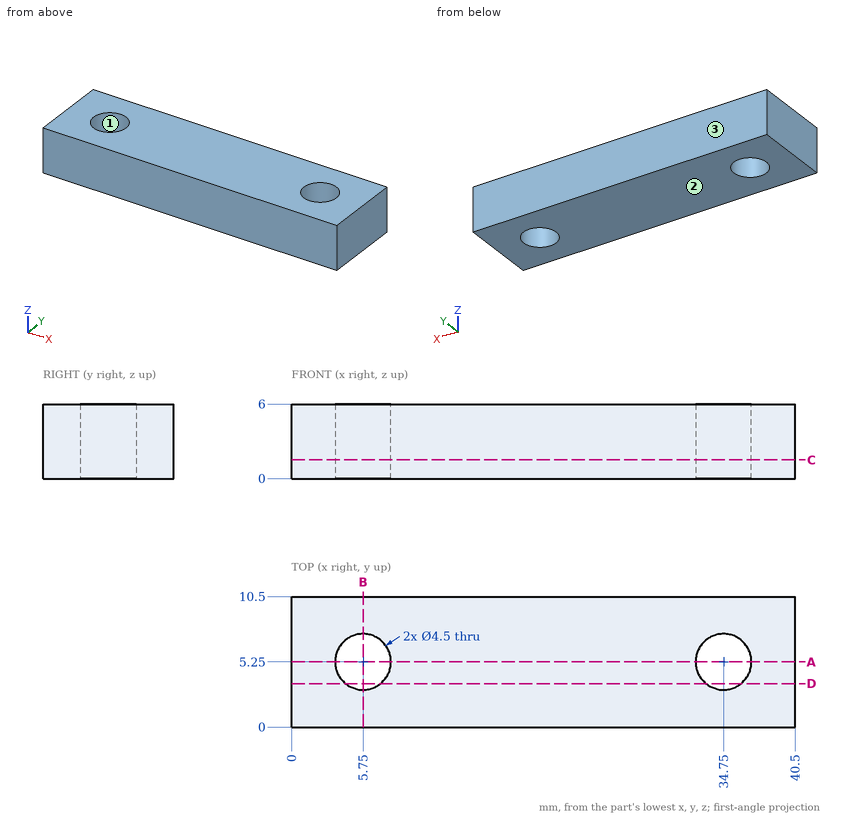
Could you check a few things on this drawing? It's one solid part, dimensions in mm from its lowest x, y, z. Coordinates: 2 decimals unless noted, no trailing zeros. Order: outer loops, then holes, each group sorted by start corner. A loop starts at its lowest first (then second) coordinate and runs counter-clockwise, first axis right, second up. Notation, with made-up numbers: (71.25, -0.75) - (85.25, -0.75) arc R16 ccw to (85.25, 28.25) - close; hole circle Ø1 at (-5.5, 37.25). An arc over 180 degrees is marked (long way). One line per question, with ' | ' between items. Start each with the question number.
1. If we section it at A-A (y = 5.25): Write out the boundary of the cut face in (x, z).
2. Please list where these lines run through material, in increasing order: line 1 along Y through (x, z) = (34.75, 1.45); line 2 along X through (y, z) = (3.5, 0.95); line 3 along X through (y, z) = (4, 2.8). Write a range as [from, to].
3. If we section it at C-C (z = 1.5): Write out the boundary of the cut face in (x, y), and give its area (3 significant figures).
4. If we section it at B-B (x = 5.75): Write out the boundary of the cut face in (y, z).
5. If we section it at D-D (y = 3.5): Write out the boundary of the cut face in (x, z), and give its area (3 significant figures).
6. I'm going to push a flat-ended pin straight in: pin 1 Ø1.5 at (x, y) = (24.5, 3.5) entering from -Z. Where does the tip first touch, or does it pass through?
7. If we mould it in two halves opening along Y, with no side actions, what happens to the marked faces 1, 2 and 3? For each: released by +Y, released by -Y, zero draft, split by the parting line, or undercut.
Model answer:
1) outline: (0, 0) - (3.5, 0) - (3.5, 6) - (0, 6) - close; (8, 0) - (32.5, 0) - (32.5, 6) - (8, 6) - close; (37, 0) - (40.5, 0) - (40.5, 6) - (37, 6) - close
2) line 1: y = [0, 3], [7.5, 10.5] | line 2: x = [0, 4.34], [7.16, 33.34], [36.16, 40.5] | line 3: x = [0, 3.88], [7.62, 32.88], [36.62, 40.5]
3) outline: (0, 0) - (40.5, 0) - (40.5, 10.5) - (0, 10.5) - close; hole circle Ø4.5 at (5.75, 5.25); hole circle Ø4.5 at (34.75, 5.25) | area: 393 mm²
4) outline: (0, 0) - (3, 0) - (3, 6) - (0, 6) - close; (7.5, 0) - (10.5, 0) - (10.5, 6) - (7.5, 6) - close
5) outline: (0, 0) - (4.34, 0) - (4.34, 6) - (0, 6) - close; (7.16, 0) - (33.34, 0) - (33.34, 6) - (7.16, 6) - close; (36.16, 0) - (40.5, 0) - (40.5, 6) - (36.16, 6) - close | area: 209 mm²
6) pin 1: stops at z = 0
7) face 1: undercut | face 2: zero draft | face 3: released by +Y
